Read the model definition and answer for the solid it produces. Units are mm, in the model's axes. A direction names the side the tool comes from. Round coordinates to 2 decimals unless told otherwise and drop trailing zeros. Order: outer loops, then holes, each group sorted by start corner. A loop starts at its lowest first (then second) coordinate and runs counter-clockwise, first axis right, second up. Notation, with made-up numbers: (-39.5, 38.5) - (1.5, 38.5) arc R19 cw to (1.5, 56.5) - close; hole circle Ø7 at (25, -19.5). An arc over 180 degrees is marked (long way). Answer as a JSON object with one key per item and string values. Group by question number.
Q1. A cutting plane is placed at D-D on z = 0.25. Determine the outline of the cut face in (x, y).
Q2. A cutting plane is placed at C-C on y = 22. Determine the outline of the cut face in (x, z), and give its area (3 significant figures).
Q3. A tool of negligible diameter and unlimited length cuts with its end or side. For faces 4 (the flat face through (-23, 3, 3.495)), 5 (the cylindrical face through (-8.65, 39.7, 0.2)), 6 (the flat face through (24, 29.5, 0)), 7 (the flat face through (-20.15, 33, 0)), from which of +Z, -Z, +X, -X, +Y, -Y can it reach the whole face along a straight path? Write none if from no direction.
Q4. Given pin 1 Ø4 at (x, z) = (20, 2.5) entering from -Y; pin 2 Ø1 at (y, z) = (25, 2) entering from -X; pin 3 Ø5 at (x, z) = (24.315, -5) entering from +Y; pin 4 Ø4 at (x, z) = (-1, 2) entering from +Y, each flat-ended and moving along its own axis, determine where each tip first touches the part or whether it passes through.
Q5. A cutting plane is placed at A-A on z = 7.75. Determine the outline of the cut face in (x, y), and give its area (3 significant figures).
Q6. The mould has two halves that part along Y. Classify faces 1 (the flat face through (-23, 5.064, 0)), 2 (the cylindrical face through (-24.4, 28.3, -3)), 3 (the flat face through (24, 27, 0)): pulls with the +Y half, pulls with the -Y half, needs draft (parallel to the pull), parting line crosses it, or undercut.
Q7. Consider line 1 (X direction, y = 39.75, z = 0) (3 decimals); line 2 (X direction, y = 28.3, z = 5) (3 decimals); line 3 (X direction, y = 6.5, z = 7). Determine where each line is inside the solid, lowest interval first.
Q8. A cutting plane is placed at B-B on x = -11. Determine the outline of the cut face in (y, z).
```python
from build123d import *

# Parameters (mm, degrees)
SKETCH_1_W          = 40.3
SKETCH_1_H          = 19.5
EXTRUDE_1_DEPTH     = 27
SKETCH_2_W          = 54
SKETCH_2_H          = 19.5
EXTRUDE_2_DEPTH     = 2.5
CUT_EXTRUDE_1_REACH = 43.162
SKETCH_3_R          = 2
SKETCH_4_W          = 40.3
SKETCH_4_H          = 19.5
EXTRUDE_3_DEPTH     = 7
SKETCH_6_R          = 2.9
SKETCH_6_R_2        = 1.5
EXTRUDE_4_DEPTH     = 6.5
SKETCH_7_R          = 5
SKETCH_7_R_2        = 2.9
EXTRUDE_5_DEPTH     = 3
SKETCH_8_W          = 6.989880398
SKETCH_8_H          = 3.148594774
EXTRUDE_6_DEPTH     = 6


with BuildPart() as part:
    # 草图1 → 凸台-拉伸1 (new body)
    with BuildSketch(Plane(origin=(0, 0, 0), x_dir=(1, 0, 0), z_dir=(0, 1, 0))):
        Rectangle(SKETCH_1_W, SKETCH_1_H)
    extrude(amount=EXTRUDE_1_DEPTH)

    # 草图2 → 凸台-拉伸2 (add)
    with BuildSketch(Plane(origin=(0, 27, 0), x_dir=(1, 0, 0), z_dir=(0, 1, 0))):
        Rectangle(SKETCH_2_W, SKETCH_2_H)
    extrude(amount=EXTRUDE_2_DEPTH)

    # 草图3 → 切除-拉伸1 (cut, up to next)
    with BuildSketch(Plane(origin=(0, 29.5, 0), x_dir=(1, 0, 0), z_dir=(0, 1, 0)), mode=Mode.PRIVATE) as cut_extrude_1_sk1:
        with Locations(Location((24.315, 5, 0), (0, 0, 270))):
            Circle(SKETCH_3_R)
    cut_extrude_1_tool1 = extrude(cut_extrude_1_sk1.sketch, amount=-CUT_EXTRUDE_1_REACH, mode=Mode.PRIVATE) & part.part
    # 草图3 → 切除-拉伸1 (cut, up to next)
    with BuildSketch(Plane(origin=(0, 29.5, 0), x_dir=(1, 0, 0), z_dir=(0, 1, 0)), mode=Mode.PRIVATE) as cut_extrude_1_sk2:
        with Locations(Location((-24.315, 5, 0), (0, 0, 90))):
            Circle(SKETCH_3_R)
    cut_extrude_1_tool2 = extrude(cut_extrude_1_sk2.sketch, amount=-CUT_EXTRUDE_1_REACH, mode=Mode.PRIVATE) & part.part
    # 草图3 → 切除-拉伸1 (cut, up to next)
    with BuildSketch(Plane(origin=(0, 29.5, 0), x_dir=(1, 0, 0), z_dir=(0, 1, 0)), mode=Mode.PRIVATE) as cut_extrude_1_sk3:
        with Locations(Location((24.315, -5, 0), (0, 0, 90))):
            Circle(SKETCH_3_R)
    cut_extrude_1_tool3 = extrude(cut_extrude_1_sk3.sketch, amount=-CUT_EXTRUDE_1_REACH, mode=Mode.PRIVATE) & part.part
    # 草图3 → 切除-拉伸1 (cut, up to next)
    with BuildSketch(Plane(origin=(0, 29.5, 0), x_dir=(1, 0, 0), z_dir=(0, 1, 0)), mode=Mode.PRIVATE) as cut_extrude_1_sk4:
        with Locations(Location((-24.315, -5, 0), (0, 0, 270))):
            Circle(SKETCH_3_R)
    cut_extrude_1_tool4 = extrude(cut_extrude_1_sk4.sketch, amount=-CUT_EXTRUDE_1_REACH, mode=Mode.PRIVATE) & part.part
    add(cut_extrude_1_tool1.solids().sort_by_distance((24.315, 29.5, -5))[0], mode=Mode.SUBTRACT)
    add(cut_extrude_1_tool2.solids().sort_by_distance((-24.315, 29.5, -5))[0], mode=Mode.SUBTRACT)
    add(cut_extrude_1_tool3.solids().sort_by_distance((24.315, 29.5, 5))[0], mode=Mode.SUBTRACT)
    add(cut_extrude_1_tool4.solids().sort_by_distance((-24.315, 29.5, 5))[0], mode=Mode.SUBTRACT)

    # 草图4 → 凸台-拉伸3 (add)
    with BuildSketch(Plane(origin=(0, 29.5, 0), x_dir=(1, 0, 0), z_dir=(0, 1, 0))):
        Rectangle(SKETCH_4_W, SKETCH_4_H)
    extrude(amount=EXTRUDE_3_DEPTH)

    # 草图6 → 凸台-拉伸4 (add)
    with BuildSketch(Plane(origin=(0, 36.5, 0), x_dir=(1, 0, 0), z_dir=(0, 1, 0))):
        with Locations(Location((-7.165, 0, 0), (0, 0, 90))):
            Circle(SKETCH_6_R)
        with Locations(Location((-7.165, 0, 0), (0, 0, 90))):
            Circle(SKETCH_6_R_2, mode=Mode.SUBTRACT)
    extrude(amount=EXTRUDE_4_DEPTH)

    # 草图7 → 凸台-拉伸5 (add)
    with BuildSketch(Plane(origin=(0, 36.5, 0), x_dir=(1, 0, 0), z_dir=(0, 1, 0))):
        with Locations(Location((-7.165, 0, 0), (0, 0, 90))):
            Circle(SKETCH_7_R)
        with Locations(Location((-7.165, 0, 0), (0, 0, 90))):
            Circle(SKETCH_7_R_2, mode=Mode.SUBTRACT)
    extrude(amount=EXTRUDE_5_DEPTH)

    # 草图8 → 凸台-拉伸6 (add)
    with BuildSketch(Plane.ZY.offset(20.15)):
        with Locations((0, 3.490037893)):
            Rectangle(SKETCH_8_W, SKETCH_8_H)
    extrude(amount=EXTRUDE_6_DEPTH)


solid = part.part
```
Result set:
{
 "1": {"outline": "(-27, 27) - (-20.15, 27) - (-20.15, 5.06) - (-26.15, 5.06) - (-26.15, 1.92) - (-20.15, 1.92) - (-20.15, 0) - (20.15, 0) - (20.15, 27) - (27, 27) - (27, 29.5) - (20.15, 29.5) - (20.15, 36.5) - (-2.17, 36.5) - (-2.17, 39.5) - (-4.28, 39.5) - (-4.28, 43) - (-5.69, 43) - (-5.69, 36.5) - (-8.64, 36.5) - (-8.64, 43) - (-10.05, 43) - (-10.05, 39.5) - (-12.16, 39.5) - (-12.16, 36.5) - (-20.15, 36.5) - (-20.15, 29.5) - (-27, 29.5) - close"},
 "2": {"outline": "(-20.15, -9.75) - (20.15, -9.75) - (20.15, 9.75) - (-20.15, 9.75) - close", "area": "786 mm²"},
 "3": {"face 4": "+Z, -X, -Y", "face 5": "+Y", "face 6": "+Z, -Z, +X, +Y", "face 7": "+Z, -Z, -X, +Y"},
 "4": {"pin 1": "stops at y = 0", "pin 2": "stops at x = -20.15", "pin 3": "stops at y = 29.5", "pin 4": "stops at y = 39.5"},
 "5": {"outline": "(-27, 27) - (-20.15, 27) - (-20.15, 0) - (20.15, 0) - (20.15, 27) - (27, 27) - (27, 29.5) - (20.15, 29.5) - (20.15, 36.5) - (-20.15, 36.5) - (-20.15, 29.5) - (-27, 29.5) - close", "area": "1,510 mm²"},
 "6": {"face 1": "undercut", "face 2": "needs draft", "face 3": "pulls with the -Y half"},
 "7": {"line 1": "x = -10.065 to -8.665, -5.665 to -4.265", "line 2": "x = -27 to -26.315, -22.315 to 22.315, 26.315 to 27", "line 3": "x = -20.15 to 20.15"},
 "8": {"outline": "(0, -9.75) - (36.5, -9.75) - (36.5, -3.21) - (39.5, -3.21) - (39.5, 3.21) - (36.5, 3.21) - (36.5, 9.75) - (0, 9.75) - close"}
}
